Work out the finished part from the listing and answer in its coordinate system (mm). Face numbers are marked on the shaded views. A direction names the side the tool comes from. Coordinates: 2 decimals unless noted, no trailing zeros. Write each loop counter-clockwise with the first axis right and the second up, starting at its lowest first coordinate (ties: lowest second). Pieces come first, ordered by that corner, then holes. Notation, with made-up numbers: (83.25, -30.5) - (118.25, -30.5) arc R14 ccw to (118.25, -16.5) - close; hole circle Ø7 at (86, 73.25). An arc over 180 degrees is marked (long way). Answer as a JSON object with one key per item and string values. Group by question number.
from build123d import *

# Parameters (mm, degrees)
SKETCH1_R               = 20
SKETCH1_R_2             = 15
BOSS_EXTRUDE1_DEPTH     = 10
BOSS_EXTRUDE2_DEPTH     = 20
SKETCH3_W               = 4
SKETCH3_H               = 31.92260483
BOSS_EXTRUDE4_DEPTH     = 20
BOSS_EXTRUDE5_DEPTH     = 20
SKETCH4_R               = 20
CUT_EXTRUDE1_DEPTH      = 11
CUT_EXTRUDE2_DEPTH      = 39
CUT_EXTRUDE3_DEPTH      = 39
SKETCH8_R               = 2
CUT_EXTRUDE4_DEPTH      = 39
FILLET4_R               = 3
SKETCH9_W               = 21.007104118
SKETCH9_H               = 10.314289307
CUT_EXTRUDE5_DEPTH      = 3
CUT_EXTRUDE5_DEPTH_BACK = 39
CUT_EXTRUDE6_DEPTH      = 19
CUT_EXTRUDE7_DEPTH      = 19
SKETCH12_R              = 4
CUT_EXTRUDE8_DEPTH      = 2
CUT_EXTRUDE9_DEPTH      = 2
BOSS_EXTRUDE7_DEPTH     = 20
SKETCH19_R              = 20.125
CUT_EXTRUDE11_DEPTH     = 11
SKETCH20_R              = 15
SKETCH20_R_2            = 12
BOSS_EXTRUDE8_DEPTH     = 10
SKETCH21_R              = 12
BOSS_EXTRUDE9_DEPTH     = 2.5
SKETCH22_R              = 10
CUT_EXTRUDE12_DEPTH     = 2.5
SKETCH23_R              = 17.5
CUT_EXTRUDE13_DEPTH     = 2.5
SKETCH24_R              = 2
CUT_EXTRUDE14_DEPTH     = 8.5


with BuildPart() as part:
    # Sketch1 → Boss-Extrude1 (new body)
    with BuildSketch(Plane.XY):
        Circle(SKETCH1_R)
        Circle(SKETCH1_R_2, mode=Mode.SUBTRACT)
    extrude(amount=BOSS_EXTRUDE1_DEPTH)

    # Sketch2 → Boss-Extrude2 (add)
    with BuildSketch(Plane.XY.offset(10)):
        with BuildLine():
            Line((2, 39.866068747), (2, 19.899748742))
            ThreePointArc((2, 19.899748742), (4.02100681, 19.591618214), (6, 19.078784028))
            Line((6, 19.078784028), (6, 39.866068747))
            Line((6, 39.866068747), (2, 39.866068747))
        make_face()
    extrude(amount=-BOSS_EXTRUDE2_DEPTH)

    # Sketch3 → Boss-Extrude4 (add)
    with BuildSketch(Plane.XY.offset(10)):
        with Locations((16, 24.679100302)):
            Rectangle(SKETCH3_W, SKETCH3_H)
    extrude(amount=-BOSS_EXTRUDE4_DEPTH)

    # Sketch5 → Boss-Extrude5 (add)
    with BuildSketch(Plane.XY.offset(10)):
        Polygon((14, 20.353512461), (10.603962903, 16.957475365), (14, 14.282856857), align=None)
    extrude(amount=-BOSS_EXTRUDE5_DEPTH)

    # Sketch4 → Cut-Extrude1 (cut, through all)
    with BuildSketch(Plane(origin=(0, 0, 0), x_dir=(-1, 0, 0), z_dir=(0, 0, -1))):
        Circle(SKETCH4_R)
    extrude(amount=CUT_EXTRUDE1_DEPTH, mode=Mode.SUBTRACT)

    # Sketch6 → Cut-Extrude2 (cut, through all)
    with BuildSketch(Plane(origin=(18, 0, 0), x_dir=(0, 0, -1), z_dir=(1, 0, 0))):
        Polygon((-10, 40.640402717), (-6, 40.640402717), (-10, 36.640402717), align=None)
    extrude(amount=-CUT_EXTRUDE2_DEPTH, mode=Mode.SUBTRACT)

    # Sketch7 → Cut-Extrude3 (cut, through all)
    with BuildSketch(Plane(origin=(18, 0, 0), x_dir=(0, 0, -1), z_dir=(1, 0, 0))):
        Polygon((10, 40.640402717), (6, 40.640402717), (10, 36.640402717), align=None)
    extrude(amount=-CUT_EXTRUDE3_DEPTH, mode=Mode.SUBTRACT)

    # Sketch8 → Cut-Extrude4 (cut, through all)
    with BuildSketch(Plane(origin=(18, 0, 0), x_dir=(0, 0, -1), z_dir=(1, 0, 0))):
        with Locations((0, 25.640402717)):
            Circle(SKETCH8_R)
    extrude(amount=-CUT_EXTRUDE4_DEPTH, mode=Mode.SUBTRACT)

    # Fillet4
    fillet4_edges = [part.edges().sort_by_distance(p)[0] for p in [
        (18, 8.717797887, 5),
    ]]
    fillet(fillet4_edges, radius=FILLET4_R)

    # Sketch9 → Cut-Extrude5 (cut, two sides)
    with BuildSketch(Plane(origin=(18, 0, 0), x_dir=(0, 0, -1), z_dir=(1, 0, 0))) as cut_extrude5_sk:
        with Locations((0.503552059, 36.79754737)):
            Rectangle(SKETCH9_W, SKETCH9_H)
    extrude(amount=CUT_EXTRUDE5_DEPTH, mode=Mode.SUBTRACT)
    extrude(cut_extrude5_sk.sketch, amount=-CUT_EXTRUDE5_DEPTH_BACK, mode=Mode.SUBTRACT)

    # Sketch10 → Cut-Extrude6 (cut, through all)
    with BuildSketch(Plane.ZY.offset(-2)):
        Polygon((10, 31.640402717), (5, 31.640402717), (10, 25.770075729), align=None)
    extrude(amount=-CUT_EXTRUDE6_DEPTH, mode=Mode.SUBTRACT)

    # Sketch11 → Cut-Extrude7 (cut, through all)
    with BuildSketch(Plane.ZY.offset(-2)):
        Polygon((-10, 31.640402717), (-10, 25.770075729), (-5, 31.640402717), align=None)
    extrude(amount=-CUT_EXTRUDE7_DEPTH, mode=Mode.SUBTRACT)

    # Sketch12 → Cut-Extrude8 (cut)
    with BuildSketch(Plane(origin=(18, 0, 0), x_dir=(0, 0, -1), z_dir=(1, 0, 0))):
        with Locations((0, 25.640402717)):
            Circle(SKETCH12_R)
    extrude(amount=-CUT_EXTRUDE8_DEPTH, mode=Mode.SUBTRACT)

    # Sketch13 → Cut-Extrude9 (cut)
    with BuildSketch(Plane.ZY.offset(-2)):
        Polygon((4.041451884, 25.640402717), (2.020725942, 29.140402717), (-2.020725942, 29.140402717), (-4.041451884, 25.640402717), (-2.020725942, 22.140402717), (2.020725942, 22.140402717), align=None)
    extrude(amount=-CUT_EXTRUDE9_DEPTH, mode=Mode.SUBTRACT)

    # Sketch16 → Boss-Extrude7 (add)
    with BuildSketch(Plane.XY.offset(10)):
        with BuildLine():
            Line((14, 20.353512461), (6, 20.353512461))
            Line((6, 20.353512461), (6, 19.078784028))
            ThreePointArc((6, 19.078784028), (8.369461371, 18.164584123), (10.603962903, 16.957475365))
            Line((10.603962903, 16.957475365), (14, 20.353512461))
        make_face()
    extrude(amount=-BOSS_EXTRUDE7_DEPTH)

    # Sketch19 → Cut-Extrude11 (cut, through all)
    with BuildSketch(Plane(origin=(0, 0, 0), x_dir=(-1, 0, 0), z_dir=(0, 0, -1))):
        Circle(SKETCH19_R)
    extrude(amount=CUT_EXTRUDE11_DEPTH, mode=Mode.SUBTRACT)

    # Sketch20 → Boss-Extrude8 (add)
    with BuildSketch(Plane.XY.offset(10)):
        Circle(SKETCH20_R)
        Circle(SKETCH20_R_2, mode=Mode.SUBTRACT)
    extrude(amount=-BOSS_EXTRUDE8_DEPTH)

    # Sketch21 → Boss-Extrude9 (add)
    with BuildSketch(Plane.XY.offset(10)):
        Circle(SKETCH21_R)
    extrude(amount=-BOSS_EXTRUDE9_DEPTH)

    # Sketch22 → Cut-Extrude12 (cut)
    with BuildSketch(Plane(origin=(0, 0, 7.5), x_dir=(-1, 0, 0), z_dir=(0, 0, -1))):
        Circle(SKETCH22_R)
    extrude(amount=-CUT_EXTRUDE12_DEPTH, mode=Mode.SUBTRACT)

    # Sketch23 → Cut-Extrude13 (cut)
    with BuildSketch(Plane(origin=(0, 0, 0), x_dir=(-1, 0, 0), z_dir=(0, 0, -1))):
        Circle(SKETCH23_R)
    extrude(amount=-CUT_EXTRUDE13_DEPTH, mode=Mode.SUBTRACT)

    # Sketch24 → Cut-Extrude14 (cut, through all)
    with BuildSketch(Plane(origin=(0, 0, 2.5), x_dir=(-1, 0, 0), z_dir=(0, 0, -1))):
        with Locations((0, 15)):
            Circle(SKETCH24_R)
        with Locations((10.606601718, 10.606601718)):
            Circle(SKETCH24_R)
        with Locations((15, 0)):
            Circle(SKETCH24_R)
        with Locations((10.606601718, -10.606601718)):
            Circle(SKETCH24_R)
        with Locations((0, -15)):
            Circle(SKETCH24_R)
        with Locations((-10.606601718, -10.606601718)):
            Circle(SKETCH24_R)
        with Locations((-15, 0)):
            Circle(SKETCH24_R)
        with Locations((-10.606601718, 10.606601718)):
            Circle(SKETCH24_R)
    extrude(amount=-CUT_EXTRUDE14_DEPTH, mode=Mode.SUBTRACT)


solid = part.part
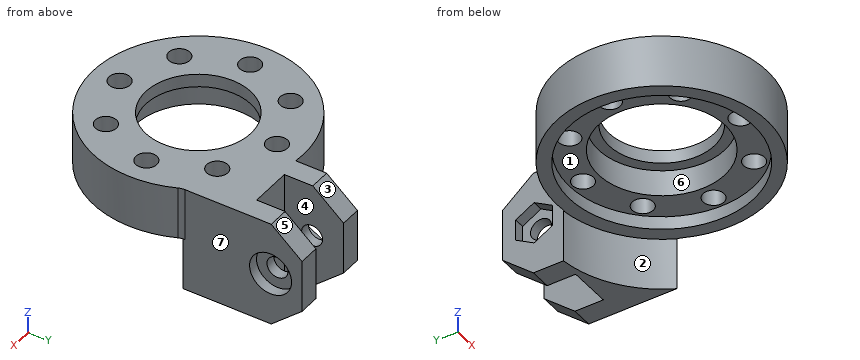
Q1. Consider L1, parallel to Y at x = 0, z = 8; L2, parallel to Y at x = 1.5, z = 6; L3, parallel to X at y = 25.5, z = -7. Determine where each line is inside the solid, lowest interval first. Write a range as from..to.
Q2. For a pull along Y with two mould halves and no side action, classify the marked faces 1, 2 and 3 as +Y half, -Y half, draft (parallel to the pull), parting line (faces both ways), or undercut.
Q3. Section B-B on x = 15 is taken. Determine the outline of the cut face in (y, z).
Q4. Section C-C on x = -15 is taken. Determine the outline of the cut face in (y, z), plus the area to 3 significant figures.
Q5. Section D-D on z = -7.5 is taken. Determine the outline of the cut face in (x, y) (3 decimals).
Q6. Section A-A on y = 15 is taken. Determine the outline of the cut face in (x, z), plus the area to 3 significant figures.
Q7. Flat-ended cylindrical pins translate along their axes: pin 1 Ø12 at (x, y) = (-14, 1.5) entering from +Z; pin 2 Ø6 at (x, y) = (-14.5, 7.5) entering from -Z; pin 3 Ø6 at (y, z) = (-12, -2) entering from +X; pin 4 Ø3 at (y, z) = (11, 6) entering from +X. Find the tip coordinate at first contact, or state that the pin passes through.
Q8. A tool of negligible diameter and unlimited length cuts with its end or side. For the marked faces 4, 5, 6 and 7, from which of +Z, -Z, +X, -X, +Y, -Y can it reach the whole face along a straight path? Write none if from no direction.
Numbers:
{
 "1": {"L1": "y = -20..-17, -13..-10, 10..13, 17..20", "L2": "y = -19.94..-16.32, -13.68..-11.91, 11.91..13.68, 16.32..19.94", "L3": "x = 2..6, 14..18"},
 "2": {"face 1": "undercut", "face 2": "-Y half", "face 3": "+Y half"},
 "3": {"outline": "(-13.23, 0) - (-9.01, 0) - (-9.01, 2.5) - (-2, 2.5) - (-2, 10) - (-13.23, 10) - close; (2, 2.5) - (9.01, 2.5) - (9.01, 0) - (13.42, 0) - (13.42, -10) - (25.77, -10) - (31.64, -5) - (31.64, 5) - (25.77, 10) - (2, 10) - close; hole circle Ø4 at (25.64, 0)"},
 "4": {"outline": "(-13.23, 0) - (-9.01, 0) - (-9.01, 2.5) - (-2, 2.5) - (-2, 10) - (-13.23, 10) - close; (2, 2.5) - (9.01, 2.5) - (9.01, 0) - (13.23, 0) - (13.23, 10) - (2, 10) - close", "area": "190 mm²"},
 "5": {"outline": "(2, 20.025) arc R20.125 cw to (18, 9.001) - (18, 28.705) - (14, 28.705) - (14, 20.354) - (6, 20.354) - (6, 28.705) - (2, 28.705) - close"},
 "6": {"outline": "(-13.23, 0) - (-9.01, 0) - (-9.01, 2.5) - (-2, 2.5) - (-2, 10) - (-13.23, 10) - close; (2, 2.5) - (9.01, 2.5) - (9.01, 0) - (13.42, 0) - (13.42, -10) - (18, -10) - (18, 10) - (2, 10) - close", "area": "283 mm²"},
 "7": {"pin 1": "stops at z = 10", "pin 2": "stops at z = 0", "pin 3": "stops at x = 17.45", "pin 4": "stops at x = 18"},
 "8": {"face 4": "+Z, -Z, +Y", "face 5": "+Z, +X, -X, +Y", "face 6": "-Z", "face 7": "+Z, -Z, +X, +Y"}
}
